Autodesk Inventor part; units mm, degrees
ref_plane "YZ Plane" through (0, 0, 0) normal (1, 0, 0) x (0, 1, 0)
ref_plane "XZ Plane" through (0, 0, 0) normal (0, 1, 0) x (-1, 0, 0)
ref_plane "XY Plane" through (0, 0, 0) normal (0, 0, 1) x (1, 0, 0)
sketch "Sketch1" plane through (0, 0, 0) normal (0, 0, 1) x (1, 0, 0)
  line L0 (0, 20) -> (0, 0)
  line L1 (0, 0) -> (20, 0)
  line L2 (20, 0) -> (20, 1)
  line L3 (20, 1) -> (1, 1)
  line L4 (1, 1) -> (1, 20)
  line L5 (1, 20) -> (0, 20)
  dimension "d0" = 20
  dimension "d1" = 20
  dimension "d2" = 1
  dimension "d3" = 1
extrude "Extrusion1" add sketch "Sketch1" along normal blind 20
sketch "Sketch2" plane through (1, 1, 0) normal (1, 0, 0) x (0, 0, -1)
  line L0 (0, 19) -> (-20, 19)
  line L1 (0, 0) -> (0, 19)
  point P0 (0, -1)
  point P1 (-10, 9.5)
  point P2 (-10, 19)
  point P3 (0, 9.5)
hole "Hole1" at (1, 10.5, 10) direction (-1, 0, 0) diameter 4.5 end through all
sketch "Sketch3" plane through (1, 1, 0) normal (0, 1, 0) x (1, 0, 0)
  line L0 (-1, 0) -> (19, 0)
  line L1 (19, 0) -> (19, -20)
  point P0 (9, -10)
  point P1 (9, 0)
  point P2 (19, -10)
hole "Hole2" at (10, 1, 10) direction (0, -1, 0) diameter 4.5 end through all
fillet "Fillet1" radius 2 1 edges at (1, 1, 10)
fillet "Fillet2" radius 10 4 edges at (0.5, 20, 20) (0.5, 20, 0) (20, 0.5, 0) (20, 0.5, 20)
fillet "Fillet3" radius 1 1 edges at (0, 0, 10)
properties part number "Vertical Support - 90deg Bracket"
The model under review builds one solid part; all positions refer to its coordinate system, in mm. A direction names the side the tool comes from. Coordinates: 2 decimals unless noted, no trailing zeros. Loops run counter-clockwise (first coordinate to the right, second up) from the corner with the lowest first, then second, coordinate; pieces in that order, holes last. Notation, with made-up numbers: M 60,18.5 L 93,18.5 A14 cw 93,25.5 Z; hole C 70,21 d1. An arc over 180 degrees is marked long. Put each result on its own line as item: value. Start each with the question number.
Q1. Add section A-A (x = 11). Write out the cut boundary in (y, z).
Q2. The part is to be moulded in two halves that separate along X. For faces 3 (the cylindrical face through (8.48, 0.49, 8.34)), 4 (the cylindrical face through (0.49, 17.15, 3.01)), 5 (the flat face through (0, 9, 8)), say which applies: +X half, -X half, draft (parallel to the pull), parting line (faces both ways), or undercut.
Q3. For faces 1 (the cylindrical face through (17.15, 0.51, 3.01)), 2 (the flat face through (1, 11.4, 7.6)), list the 3-axis set-ups (+Z, -Z, +X, -X, +Y, -Y) from which the entire face can be reached by the end or side of a thin tool; tool diameter is ignored.
Q4. Add section C-C (y = 10.5). Write out the cut boundary in (x, z).
Q5. Clearance check with flat-ended pins moving along their axes: pin 1 (3 mm diameter, centred on x = 16, z = 15, fed in from +Y); pin 2 (7 mm diameter, centred on y = 10.5, z = 10, fed in from +X); pin 3 (2 mm diameter, centred on x = 2.5, z = 2.5, fed in from +Y). State where each tip first meets the part, or that it passes through.
Q6. Add section B-B (z = 9.5). Write out the cut boundary in (x, y).
Q7. Add section D-D (z = 3). Write out the cut boundary in (x, y).
Q8. Wall thickness on line 1 (Z direction, x = 10, y = 0.7); line 2 (X direction, y = 16, z = 16): over which ranges is each line inside the solid? List them lowest first.
Answers:
1. outline: M 0,0.05 L 1,0.05 L 1,7.98 L 0,7.98 Z; M 0,12.02 L 1,12.02 L 1,19.95 L 0,19.95 Z
2. face 3: undercut
2. face 4: draft
2. face 5: -X half
3. face 1: -Z, +X, +Y, -Y
3. face 2: +Z, -Z, +X, +Y
4. outline: M 0,0.01 L 1,0.01 L 1,7.75 L 0,7.75 Z; M 0,12.25 L 1,12.25 L 1,19.99 L 0,19.99 Z
5. pin 1: stops at y = 1
5. pin 2: stops at x = 1
5. pin 3: stops at y = 1.68
6. outline: M 0,1 A1 ccw 1,0 L 7.81,0 L 7.81,1 L 3,1 A2 cw 1,3 L 1,8.31 L 0,8.31 Z; M 0,12.69 L 1,12.69 L 1,19.99 L 0,19.99 Z; M 12.19,0 L 19.99,0 L 19.99,1 L 12.19,1 Z
7. outline: M 0,1 A1 ccw 1,0 L 17.14,0 L 17.14,1 L 3,1 A2 cw 1,3 L 1,17.14 L 0,17.14 Z
8. line 1: z = 0 to 7.75, 12.25 to 20
8. line 2: x = 0 to 1
